Check sheet for the modelled part. Datum: model origin and axes. Units: mm. Face numbers are marked on the shaded views. Round coordinates to 2 decimals unless told otherwise and drop trailing zeros. Write each loop counter-clockwise with the first axis right and the second up, starting at its lowest first coordinate (ties: lowest second). Pieces come first, ordered by that corner, then holes. Notation, with made-up numbers: (6, -12) - (13, -12) arc R14 ccw to (13, 10) - close; hole circle Ø8 at (9.5, -36.75). An arc over 180 degrees is marked (long way). Use one line per item in the form item = value. Start each with the question number.
1) Scan lines: probe 1 along Z at (x, y) = (0, -4.75) (3 decimals); probe 2 along Z at (x, y) = (0, -2.75); probe 3 along Z at (x, y) = (0, -12.5). Record each from-to range of solid material in increasing order.
2) Section check B-B (x = 0). Record the boundary of the cut face in (y, z) (3 decimals).
3) Section check A-A (y = -4.5). Record the boundary of the cut face in (x, z) (3 decimals), then the cut area to 3 significant figures.
4) Section check C-C (z = 12). Record the boundary of the cut face in (x, y).
5) Gauge pin test, flat ends, axial feed: P1, Ø3.5, axis at x = -0.5, y = -7, coming from the +Z side; P2, Ø2.5, axis at x = 0, z = 1.5, coming from the -Y side; P3, Ø8, axis at x = 2, z = 1, coming from the -Y side. Record the tip position at first contact, or that the pin passes through.
6) Draft check along Z on the marked faces 1, 2 and 3. Enter one of: +Z half, -Z half, draft (parallel to the pull), parting line (faces both ways), or undercut.
7) Section check D-D (y = -13.25). Record the boundary of the cut face in (x, z), then the cut area to 3 significant figures.
from build123d import *

# Parameters (mm, degrees)
F0_R     = 18.54
F1_DEPTH = 15
F2_R     = 17.1
F3_DEPTH = 11
F5_R     = 4.535
F6_DEPTH = 6
F9_DEPTH = 9.01


with BuildPart() as f1:
    # F0 (on Front) → F1 (new body)
    with BuildSketch(Plane.XZ):
        Circle(F0_R)
        with BuildLine():
            ThreePointArc((-2.5, -3.783679), (-2.148107, 3.993978), (4.535, 0))
            ThreePointArc((4.535, 0), (3.993978, -2.148107), (2.5, -3.783679))
            ThreePointArc((2.5, -3.783679), (0, -4.535), (-2.5, -3.783679))
        make_face(mode=Mode.SUBTRACT)
        with BuildLine():
            ThreePointArc((2.5, -3.783679), (3.993978, -2.148107), (4.535, 0))
            ThreePointArc((4.535, 0), (-2.148107, 3.993978), (-2.5, -3.783679))
            Line((-2.5, -3.783679), (2.5, -3.783679))
        make_face()
        with BuildLine():
            Line((2.5, -3.783679), (-2.5, -3.783679))
            ThreePointArc((-2.5, -3.783679), (0, -4.535), (2.5, -3.783679))
        make_face()
    extrude(amount=F1_DEPTH)

    # F2 (on face) → F3 (cut)
    with BuildSketch(Plane.XZ.offset(15)):
        Circle(F2_R)
    extrude(amount=-F3_DEPTH, mode=Mode.SUBTRACT)

    # F5 (on face) → F6 (join)
    with BuildSketch(Plane.XZ.offset(4)):
        Circle(F5_R)
    extrude(amount=F6_DEPTH)

    # F8 (on face) → F9 (cut)
    with BuildSketch(Plane.XZ.offset(10)):
        with BuildLine():
            ThreePointArc((1.662322, -3.417117), (3.221554, -2.015338), (3.8, 0))
            ThreePointArc((3.8, 0), (-2.015338, 3.221554), (-1.662322, -3.417117))
            Line((-1.662322, -3.417117), (1.662322, -3.417117))
        make_face()
    extrude(amount=-F9_DEPTH, mode=Mode.SUBTRACT)


solid = f1.part
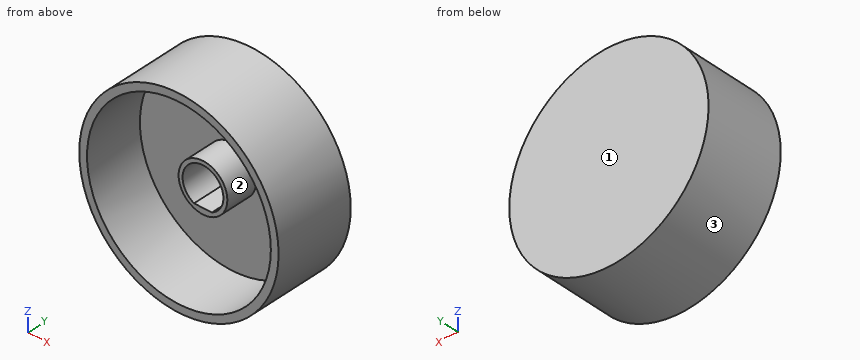
Results are:
q1.probe_1 = -18.54 to -17.1, -4.535 to -3.417, 3.8 to 4.535, 17.1 to 18.54
q1.probe_2 = -18.54 to -3.42, 3.8 to 18.54
q1.probe_3 = -18.54 to -17.1, 17.1 to 18.54
q2.outline = (-15, -18.54) - (0, -18.54) - (0, 18.54) - (-15, 18.54) - (-15, 17.1) - (-4, 17.1) - (-4, 4.535) - (-10, 4.535) - (-10, 3.8) - (-0.99, 3.8) - (-0.99, -3.417) - (-10, -3.417) - (-10, -4.535) - (-4, -4.535) - (-4, -17.1) - (-15, -17.1) - close
q3.outline = circle Ø37.08 at (0, 0); circle Ø9.07 at (0, 0); hole circle Ø34.2 at (0, 0); hole (-1.662, -3.417) - (1.662, -3.417) arc R3.8 ccw to (3.8, 0) arc R3.8 ccw (long way) to start
q3.area = 181 mm²
q4.outline = (-14.13, -15) - (-12.18, -15) - (-12.18, -4) - (12.18, -4) - (12.18, -15) - (14.13, -15) - (14.13, 0) - (-14.13, 0) - close
q5.P1 = 18.54
q5.P2 = -0.99
q5.P3 = -10
q6.face_1 = draft
q6.face_2 = undercut
q6.face_3 = parting line
q7.outline = circle Ø37.08 at (0, 0); hole circle Ø34.2 at (0, 0)
q7.area = 161 mm²
